from build123d import *

# Parameters (mm, degrees)
BOSS_EXTRUDE1_DEPTH = 35
BOSS_EXTRUDE2_DEPTH = 10
SKETCH4_W           = 35.357177314
SKETCH4_H           = 3.5
CUT_EXTRUDE1_DEPTH  = 10
SKETCH5_W           = 68.753729038
SKETCH5_H           = 5
CUT_EXTRUDE2_DEPTH  = 0.625
CUT_EXTRUDE3_REACH  = 165.362
SKETCH6_R           = 1.9
SKETCH7_R           = 3.35
CUT_EXTRUDE4_DEPTH  = 2.5
LPATTERN1_COUNT     = 2
LPATTERN1_PITCH     = 52.5
SKETCH8_W           = 3.5
SKETCH8_H           = 145
SKETCH8_W_2         = 3.25
CUT_EXTRUDE5_DEPTH  = 10
SKETCH10_W          = 40
SKETCH10_H          = 55
CUT_EXTRUDE6_DEPTH  = 5
CUT_EXTRUDE7_REACH  = 178.378
SKETCH9_W           = 13
SKETCH9_H           = 28.5
SKETCH11_W          = 17
SKETCH11_H          = 32.5
SKETCH11_W_2        = 13
SKETCH11_H_2        = 28.5
CUT_EXTRUDE8_DEPTH  = 7.5
CHAMFER1_SIZE2      = 1
CHAMFER1_SIZE       = 5
SKETCH14_W          = 25
SKETCH14_H          = 14.5
BOSS_EXTRUDE3_DEPTH = 2.5
SKETCH13_R          = 2.4
CUT_EXTRUDE9_DEPTH  = 3.8


with BuildPart() as part:
    # Sketch1 → Boss-Extrude1 (new body)
    with BuildSketch(Plane(origin=(0, 0, 0), x_dir=(-1, 0, 0), z_dir=(0, 1, 0))):
        Polygon((66.563657866, 147.59508075), (16.563657866, 147.59508075), (26.356262061, 145.56902471), (24.706480552, 137.59508075), (66.563657866, 137.59508075), align=None)
        Polygon((26.356262061, 145.56902471), (16.563657866, 147.59508075), (16.563657866, 137.59508075), (24.706480552, 137.59508075), align=None)
        Polygon((16.563657866, 147.59508075), (-13.436342134, 2.59508075), (-8.436342134, 2.59508075), (-3.224553931, 2.59508075), (-3.224553931, 7.59508075), (-2.190071172, 7.59508075), (24.706480552, 137.59508075), (16.563657866, 137.59508075), align=None)
        Polygon((76.563657866, 147.59508075), (66.563657866, 147.59508075), (66.563657866, 137.59508075), (66.563657866, 7.59508075), (66.563657866, 2.59508075), (76.563657866, 2.59508075), align=None)
        Polygon((-3.224553931, 7.59508075), (-3.224553931, 2.59508075), (-2.190071172, 7.59508075), align=None)
        Polygon((-2.190071172, 7.59508075), (-3.224553931, 2.59508075), (66.563657866, 2.59508075), (66.563657866, 7.59508075), align=None)
    extrude(amount=BOSS_EXTRUDE1_DEPTH)

    # Sketch3 → Boss-Extrude2 (add)
    with BuildSketch(Plane.XZ):
        Polygon((-76.563657866, 147.59508075), (-16.563657866, 147.59508075), (13.436342134, 2.59508075), (-76.563657866, 2.59508075), align=None)
    extrude(amount=-BOSS_EXTRUDE2_DEPTH)

    # Sketch4 → Cut-Extrude1 (cut)
    with BuildSketch(Plane(origin=(0, 35, 0), x_dir=(-1, 0, 0), z_dir=(0, 1, 0))):
        Polygon((20.865415976, 135.0709526), (-5.748682081, 6.436145326), (-9.176093549, 7.145264941), (17.438004507, 135.780072214), align=None)
        with Locations((45.635069209, 142.59508075)):
            Rectangle(SKETCH4_W, SKETCH4_H)
    extrude(amount=-CUT_EXTRUDE1_DEPTH, mode=Mode.SUBTRACT)

    # Sketch5 → Cut-Extrude2 (cut)
    with BuildSketch(Plane(origin=(0, 35, -3.02991925), x_dir=(1, 0, 0), z_dir=(0, -1, 0))):
        Polygon((3.224553931, 5.625), (2.190071172, 10.625), (2.190071172, 5.625), align=None)
        with Locations((-32.186793347, 8.125)):
            Rectangle(SKETCH5_W, SKETCH5_H)
    extrude(amount=CUT_EXTRUDE2_DEPTH, mode=Mode.SUBTRACT)

    # Sketch6 → Cut-Extrude3 (cut, up to next)
    with BuildSketch(Plane.XY.offset(7.59508075), mode=Mode.PRIVATE) as cut_extrude3_sk1:
        with Locations((-59.313657866, 29.375)):
            Circle(SKETCH6_R)
    cut_extrude3_tool1 = extrude(cut_extrude3_sk1.sketch, amount=-CUT_EXTRUDE3_REACH, mode=Mode.PRIVATE) & part.part
    cut_extrude3 = cut_extrude3_tool1.solids().sort_by_distance((-59.313658, 29.375, 7.595081))[0]
    add(cut_extrude3, mode=Mode.SUBTRACT)

    # Sketch7 → Cut-Extrude4 (cut)
    with BuildSketch(Plane.XY.offset(7.59508075)):
        with Locations((-59.313657866, 29.375)):
            Circle(SKETCH7_R)
    cut_extrude4 = extrude(amount=-CUT_EXTRUDE4_DEPTH, mode=Mode.SUBTRACT)

    # LPattern1: Cut-Extrude3, Cut-Extrude4 ×2
    with Locations(*[(i * LPATTERN1_PITCH, 0, 0) for i in range(1, LPATTERN1_COUNT)]):
        add(cut_extrude3, mode=Mode.SUBTRACT)
        add(cut_extrude4, mode=Mode.SUBTRACT)

    # Sketch8 → Cut-Extrude5 (cut)
    with BuildSketch(Plane(origin=(0, 35, 0), x_dir=(-1, 0, 0), z_dir=(0, 1, 0))):
        with Locations((71.563657866, 75.09508075)):
            Rectangle(SKETCH8_W, SKETCH8_H)
        with Locations((74.938657866, 75.09508075)):
            Rectangle(SKETCH8_W_2, SKETCH8_H)
    extrude(amount=-CUT_EXTRUDE5_DEPTH, mode=Mode.SUBTRACT)

    # Sketch10 → Cut-Extrude6 (cut)
    with BuildSketch(Plane(origin=(0, 10, 0), x_dir=(-1, 0, 0), z_dir=(0, 1, 0))):
        Polygon((15.184347521, 7.59508075), (26.563657866, 7.59508075), (26.563657866, 62.59508075), align=None)
        with Locations((46.563657866, 35.09508075)):
            Rectangle(SKETCH10_W, SKETCH10_H)
    extrude(amount=-CUT_EXTRUDE6_DEPTH, mode=Mode.SUBTRACT)

    # Sketch9 → Cut-Extrude7 (cut, up to next)
    with BuildSketch(Plane(origin=(-76.563657866, 0, 0), x_dir=(0, -1, 0), z_dir=(-1, 0, 0)), mode=Mode.PRIVATE) as cut_extrude7_sk1:
        with Locations((-12.5, 31.84508075)):
            Rectangle(SKETCH9_W, SKETCH9_H)
    cut_extrude7_tool1 = extrude(cut_extrude7_sk1.sketch, amount=-CUT_EXTRUDE7_REACH, mode=Mode.PRIVATE) & part.part
    add(cut_extrude7_tool1.solids().sort_by_distance((-76.563658, 12.5, 31.845081))[0], mode=Mode.SUBTRACT)

    # Sketch11 → Cut-Extrude8 (cut)
    with BuildSketch(Plane.YZ.offset(-66.563657866)):
        with Locations((12.5, 31.84508075)):
            Rectangle(SKETCH11_W, SKETCH11_H)
        with Locations((12.5, 31.84508075)):
            Rectangle(SKETCH11_W_2, SKETCH11_H_2, mode=Mode.SUBTRACT)
    extrude(amount=-CUT_EXTRUDE8_DEPTH, mode=Mode.SUBTRACT)

    # Chamfer1
    chamfer1_edges = [part.edges().sort_by_distance(p)[0] for p in [
        (-66.563657866, 5, 31.84508075),
    ]]
    chamfer1_side = [part.faces().sort_by_distance(p)[0] for p in [
        (-66.543657866, 5, 31.84508075),
    ]]
    chamfer(chamfer1_edges, length=CHAMFER1_SIZE - 0.0001, length2=CHAMFER1_SIZE2 - 0.0001, reference=chamfer1_side[0])  # a hair under: the kernel refuses the full size

    # Sketch14 → Boss-Extrude3 (add)
    with BuildSketch(Plane.YZ.offset(-66.563657866)):
        with Locations((22.5, 130.34508075)):
            Rectangle(SKETCH14_W, SKETCH14_H)
    extrude(amount=BOSS_EXTRUDE3_DEPTH)

    # Sketch13 → Cut-Extrude9 (cut)
    with BuildSketch(Plane(origin=(-69.813657866, 0, 0), x_dir=(0, -1, 0), z_dir=(-1, 0, 0))):
        with Locations(Location((-30, 130.34508075, 0), (0, 0, 90))):
            Circle(SKETCH13_R)
    extrude(amount=-CUT_EXTRUDE9_DEPTH, mode=Mode.SUBTRACT)


solid = part.part
The model under review builds one solid part; all positions refer to its coordinate system, in mm. A direction names the side the tool comes from. Coordinates: 2 decimals unless noted, no trailing zeros. Write each loop counter-clockwise with the first axis right and the second up, starting at its lowest first coordinate (ties: lowest second). Pieces come first, ordered by that corner, then holes. Notation, with made-up numbers: (2, 35.25) - (26, 35.25) arc R16 cw to (26, 47.25) - close; hole circle Ø11 at (-38, 47.5). An arc over 180 degrees is marked (long way). Answer as a JSON object with one key per item and string values. Group by question number.
1. Add section C-C (x = -43). Give the boundary of the cut face in (y, z) (3 decimals).
2. Add section D-D (z = 64.5). Give the boundary of the cut face in (x, y), plus the area to 3 significant figures.
3. Mouldability with a two-part tool opening along Z and no side actions: class faces 5 (the face through (-1.774, 17.255, 76.11)), 6 (the face through (-31, 17, 2.595)), 7 (the face through (-32, 10, 88)), 8 (the face through (-13, 35, 91)) as pulls with the +Z half, pulls with the -Z half, needs draft (parallel to the pull), parting line crosses it, or undercut.
4. Machinability: for faces 1 (the face through (-74.064, 5.5, 30.7)), 2 (the face through (-64.064, 22, 130)), 3 (the face through (-7.06, 31.26, 3.86)), 4 (the face through (-67.94, 28.54, 128.44)), which of the approach directions +Z, -Z, +X, -X, +Y, -Y give a long, thin tool a straight path to every point of the face, cutting with its end or side? Answer none if there is none.
5. To check wall thickness, follow probe 1 along Z at (x, y) = (-33, 6); probe 2 along Z at (x, y) = (-70, 13.5); probe 3 along X at (y, z) = (25.5, 112.5). State the ranges of each line that lie inside material, in increasing order.
6. Add section A-A (y = 16). Give the boundary of the cut face in (x, z).
7. Clearance check with flat-ended pins moving along their axes: pin 1 Ø5.5 at (y, z) = (30, 130.35) entering from -X; pin 2 Ø1 at (y, z) = (3.5, 22.5) entering from +X; pin 3 Ø12 at (x, z) = (-52, 72.5) entering from +Y. State where each tip first meets the part, or that it passes through.
Findings:
{
 "1": {"outline": "(0, 2.595) - (34.375, 2.595) - (34.375, 7.595) - (5, 7.595) - (5, 62.595) - (10, 62.595) - (10, 137.595) - (35, 137.595) - (35, 140.845) - (25, 140.845) - (25, 144.345) - (35, 144.345) - (35, 147.595) - (0, 147.595) - close"},
 "2": {"outline": "(-76.56, 0) - (0.63, 0) - (0.63, 35) - (-2.69, 35) - (-2.69, 25) - (-6.26, 25) - (-6.26, 35) - (-9.58, 35) - (-9.58, 10) - (-66.56, 10) - (-66.56, 35) - (-69.81, 35) - (-69.81, 25) - (-76.56, 25) - close", "area": "1,170 mm²"},
 "3": {"face 5": "pulls with the +Z half", "face 6": "pulls with the -Z half", "face 7": "undercut", "face 8": "needs draft"},
 "4": {"face 1": "none", "face 2": "+Y", "face 3": "-Z", "face 4": "-X"},
 "5": {"probe 1": "2.6 to 7.6, 62.6 to 147.6", "probe 2": "2.6 to 15.6, 48.1 to 147.6", "probe 3": "-69.81 to -66.56, -19.51 to -16.2, -12.62 to -9.3"},
 "6": {"outline": "(-76.56, 2.6) - (13.44, 2.6) - (-16.56, 147.6) - (-76.56, 147.6) - (-76.56, 46.1) - (-74.06, 46.1) - (-74.06, 48.1) - (-66.56, 48.1) - (-66.56, 123.1) - (-64.06, 123.1) - (-64.06, 137.6) - (-24.71, 137.6) - (2.19, 7.6) - (-66.56, 7.6) - (-66.56, 15.6) - (-74.06, 15.6) - (-74.06, 17.6) - (-76.56, 17.6) - close"},
 "7": {"pin 1": "x = -69.81", "pin 2": "x = 9.42", "pin 3": "y = 10"}
}
